CAD build for the part. Positions are in the model's coordinates, mm. Round coordinates to 2 decimals unless told otherwise and drop trailing zeros. Loops run counter-clockwise (first coordinate to the right, second up) from the corner with the lowest first, then second, coordinate; pieces in that order, holes last. Notation, with made-up numbers: M -19.75,40 L -10.75,40 A12 cw -10.75,60 Z; hole C -4.5,-17 d5. An arc over 180 degrees is marked long. Use one line per item in the form item = value.
from build123d import *

# Parameters (mm, degrees)
F0_W     = 424.019751
F0_H     = 50.8
F1_DEPTH = 3.175
F2_W     = 57.9247
F2_H     = 5.08
F2_W_2   = 115.8494
F2_H_2   = 3.1496
F3_DEPTH = 3.175
F5_DEPTH = 3.175
F6_DEPTH = 3.176


with BuildPart() as f1:
    # F0 (on Front) → F1 (new body)
    with BuildSketch(Plane.XZ):
        with Locations((212.009875, 25.4)):
            Rectangle(F0_W, F0_H)
    extrude(amount=F1_DEPTH)

    # F2 (on face) → F3 (join)
    with BuildSketch(Plane.XZ.offset(3.175)):
        with Locations((28.96235, 53.34)):
            Rectangle(F2_W, F2_H)
        with Locations((139.123344, 53.34)):
            Rectangle(F2_W_2, F2_H)
        with Locations((284.896408, 53.34)):
            Rectangle(F2_W_2, F2_H)
        with Locations((395.057401, 53.34)):
            Rectangle(F2_W, F2_H)
        with Locations((28.96235, -1.5748)):
            Rectangle(F2_W, F2_H_2)
        with Locations((139.123344, -1.5748)):
            Rectangle(F2_W_2, F2_H_2)
        with Locations((284.896408, -1.5748)):
            Rectangle(F2_W_2, F2_H_2)
        with Locations((395.057401, -1.5748)):
            Rectangle(F2_W, F2_H_2)
    extrude(amount=-F3_DEPTH)

    # F4 (on face) → F5 (join)
    with BuildSketch(Plane.XZ.offset(3.175)):
        Polygon((0, 7.3152), (0, 45.4152), (-3.175, 45.4152), (-6.35, 48.5902), (-6.35, 4.1402), (-3.175, 7.3152), align=None)
    extrude(amount=-F5_DEPTH)

    # F4 (on face) → F6 (cut, through all)
    with BuildSketch(Plane.XZ.offset(3.175)):
        Polygon((424.019751, 7.3152), (424.019751, 45.4152), (420.844751, 45.4152), (417.669751, 48.5902), (417.669751, 4.1402), (420.844751, 7.3152), align=None)
    extrude(amount=-F6_DEPTH, mode=Mode.SUBTRACT)


solid = f1.part
1. Drop flat-ended pins along their axis: P1, Ø1.6, axis at y = -1.5, z = 2, coming from the -X side; P2, Ø1, axis at x = 206.5, y = -1.5, coming from the +Z side; P3, Ø1, axis at x = 349, y = -2, coming from the -Z side. Give the stop position or say it passes through.
Completed:
P1 = 0
P2 = 50.8
P3 = 0
2. Cut at A-A on x = 216. Write the cut outline in (y, z) (3 decimals).
Completed:
outline = M -3.175,0 L 0,0 L 0,50.8 L -3.175,50.8 Z
3. Probe line 1 along X through (y, z) = (-0.3, 7); line 2 along X through (y, z) = (-1.6, 45); line 3 along X through (y, z) = (-1.6, 47.5). List the from-to ranges inside material, lowest first. Write a range as from..to.
Completed:
line_1 = -6.35..-3.49, 0..417.67, 420.53..424.02
line_2 = -6.35..417.67
line_3 = -6.35..-5.26, 0..417.67, 418.76..424.02
